The model under review builds one solid part; all positions refer to its coordinate system, in mm. Face numbers are marked on the shaded views. Round coordinates to 2 decimals unless told otherwise and drop trailing zeros. Order: outer loops, then holes, each group sorted by start corner. A loop starts at its lowest first (then second) coordinate and runs counter-clockwise, first axis right, second up. Notation, with made-up numbers: (73, 11.5) - (126, 11.5) arc R19 ccw to (126, 18.5) - close; hole circle Ø2 at (25, -6.75). An arc over 180 degrees is marked (long way). One line per question, with ' | ' between items. Start each with the question number.
Item 1: Add section A-A on x = -24.5. State the section outline as (y, z) points, and give its area (3 significant figures).
Item 2: Insertion check: pin 1 Ø6 at (y, z) = (19, 5.5) entering from -X. The pin has a flat end and moves straight along its axis. Give the tip position at first contact, or say it passes through.
Item 3: Add section B-B on y = 17.25. State how many separate pieces and enclosed holes the cut face has, and give its area (3 significant figures).
Item 4: Add section C-C on x = 11.5. State the section outline as (y, z) points.
Item 5: For L1, parallel to X at y = 22.5, z = 5 (3 decimals); L2, parallel to X at y = 23, z = 5.5; L3, parallel to Z at x = -24.5, y = 18, list the stretches that pass through material, from the lowest coordinate up. Write a range as [from, to].
Item 6: Draft analysis for pull direction X (two halves, no side actions). For the marked faces 1, 2 and 3, state which applies: +X half, -X half, draft (parallel to the pull), parting line (faces both ways), or undercut.
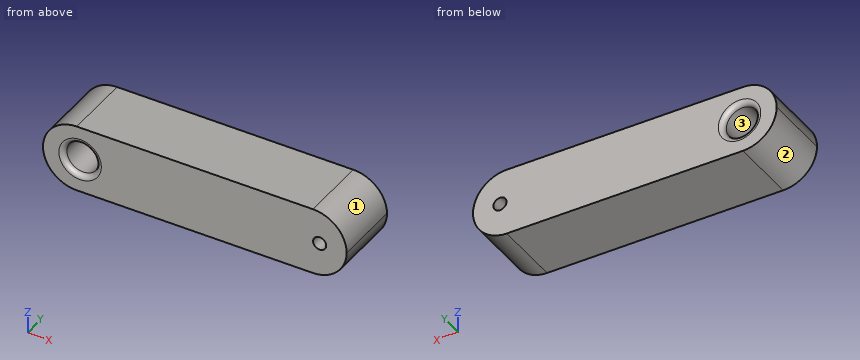
Autodesk Fusion 360 part; units mm, degrees
sketch "Esquisse1" plane through (0, 0, 0) normal (0, 0, 1) x (1, 0, 0)
  line L0 (-30, 25) -> (15, 25)
  line L1 (15, 25) -> (15, 15)
  line L2 (15, 15) -> (-30, 15)
  line L3 (-30, 15) -> (-30, 25)
  dimension "d21" = 10
  dimension "d22" = 45
extrude "Extrusion1" add sketch "Esquisse1" along normal blind 10
sketch "Esquisse2" plane through (0, 0, 0) normal (0, 1, 0) x (1, 0, 0)
  circle A0 centre (-24.5, -5) radius 2.4
  circle A1 centre (11, -5) radius 0.975
  line L0 (15, 0) -> (15, -10)
  line L1 (-30, 0) -> (-30, -10)
  dimension "d3" = 4.8
  dimension "d4" = 1.95
  dimension "d25" = 4
  dimension "d26" = 5.5
extrude "Extrusion2" cut sketch "Esquisse2" along normal blind 25 and the other way blind -15
fillet "Congé4" radius 5 4 edges at (-30, 20, 10) (15, 20, 10) (15, 20, 0) (-30, 20, 0)
fillet "Congé5" radius 0.75 2 edges at (-26.7376, 15, 5.8679) (-26.7376, 25, 4.1321)
Determined:
1) outline: (15, 0) - (25, 0) - (25, 1.85) arc R0.75 ccw to (24.25, 2.6) - (15.75, 2.6) arc R0.75 ccw to (15, 1.85) - close; (15, 8.15) arc R0.75 ccw to (15.75, 7.4) - (24.25, 7.4) arc R0.75 ccw to (25, 8.15) - (25, 10) - (15, 10) - close | area: 51.5 mm2
2) pin 1: x = -30
3) separate pieces: 1 | enclosed holes: 2 | area: 407 mm2
4) outline: (15, 0.23) - (25, 0.23) - (25, 4.16) - (15, 4.16) - close; (15, 5.84) - (25, 5.84) - (25, 9.77) - (15, 9.77) - close
5) L1: [-30, -26.9], [-22.1, 10.025], [11.975, 15] | L2: [-29.98, -26.85], [-22.15, 10.16], [11.84, 14.98] | L3: [0, 2.6], [7.4, 10]
6) face 1: +X half | face 2: -X half | face 3: undercut
